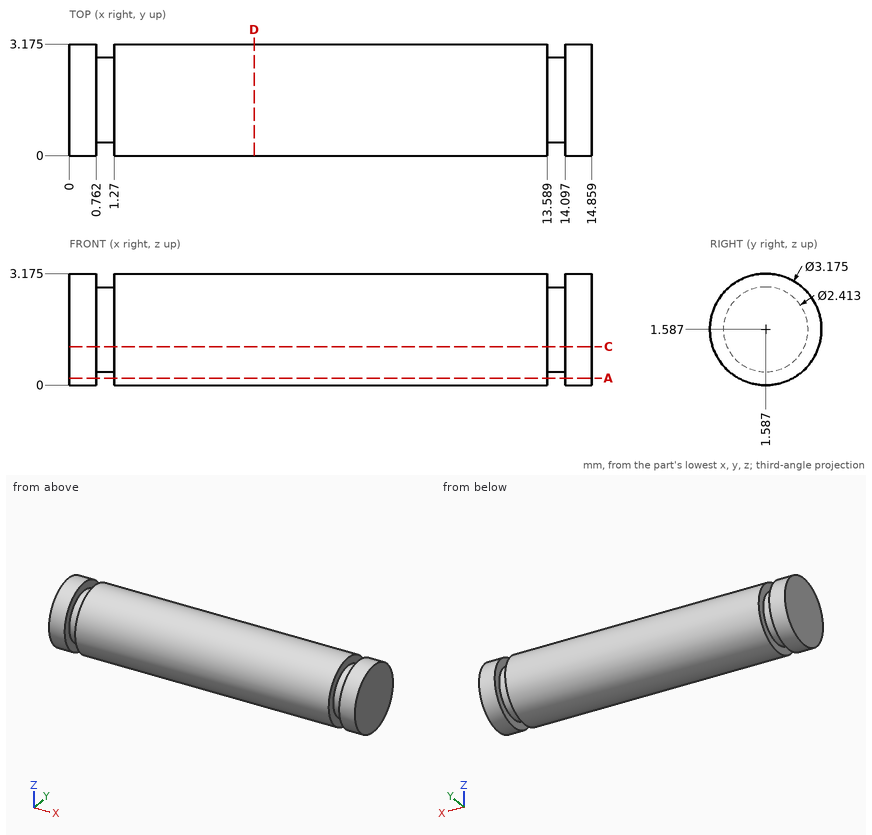
Study the drawing (mm; zero at the part's minimum x, y, z) and answer. Round coordinates to 2 decimals unless told otherwise and drop trailing zeros. Loops run counter-clockwise (first coordinate to the right, second up) from the corner with the lowest first, then second, coordinate; pieces in that order, holes last. Notation, with made-up numbers: (18, -4.5) -> (47, -4.5) arc R20 ccw to (47, 16.5) -> close; hole circle Ø9 at (-35.5, 13). An arc over 180 degrees is marked (long way). One line per item, written item: value.
1) A cutting plane is placed at C-C (z = 1.1). Determine the outline of the cut face in (x, y).
Answer list:
outline: (0, 0.08) -> (0.76, 0.08) -> (0.76, 0.48) -> (1.27, 0.48) -> (1.27, 0.08) -> (13.59, 0.08) -> (13.59, 0.48) -> (14.1, 0.48) -> (14.1, 0.08) -> (14.86, 0.08) -> (14.86, 3.1) -> (14.1, 3.1) -> (14.1, 2.69) -> (13.59, 2.69) -> (13.59, 3.1) -> (1.27, 3.1) -> (1.27, 2.69) -> (0.76, 2.69) -> (0.76, 3.1) -> (0, 3.1) -> close
2) Consider L1, parallel to X at y = 0.3, z = 1.95; L2, parallel to Y at x = 13, z = 1.65; L3, parallel to Y at x = 10.5, z = 0.85 (1 decimal). Determine where each line is inside the solid, lowest interval first. Write a range as [from, to].
Answer list:
L1: x = [0, 0.76], [1.27, 13.59], [14.1, 14.86]
L2: y = [0, 3.17]
L3: y = [0.2, 3]
3) A cutting plane is placed at A-A (z = 0.2). Determine the outline of the cut face in (x, y).
Answer list:
outline: (0, 0.82) -> (0.76, 0.82) -> (0.76, 2.36) -> (0, 2.36) -> close; (1.27, 0.82) -> (13.59, 0.82) -> (13.59, 2.36) -> (1.27, 2.36) -> close; (14.1, 0.82) -> (14.86, 0.82) -> (14.86, 2.36) -> (14.1, 2.36) -> close
4) A cutting plane is placed at D-D (x = 5.25). Determine the outline of the cut face in (y, z) (1 decimal).
Answer list:
outline: circle Ø3.2 at (1.6, 1.6)
5) A flat-ended cylindrical pin translates along its axis: P1, Ø1.6, axis at y = 2, z = 2, coming from the -X side. Find the tip coordinate at first contact, or state that the pin passes through.
Answer list:
P1: stops at x = 0
